Could you check a few things on this drawing? It's one solid part, dimensions in mm from its lowest x, y, z. Coordinates: 2 decimals unless noted, no trailing zeros. Order: outer loops, then holes, each group sorted by start corner. A loop starts at its lowest first (then second) coordinate and runs counter-clockwise, first axis right, second up.
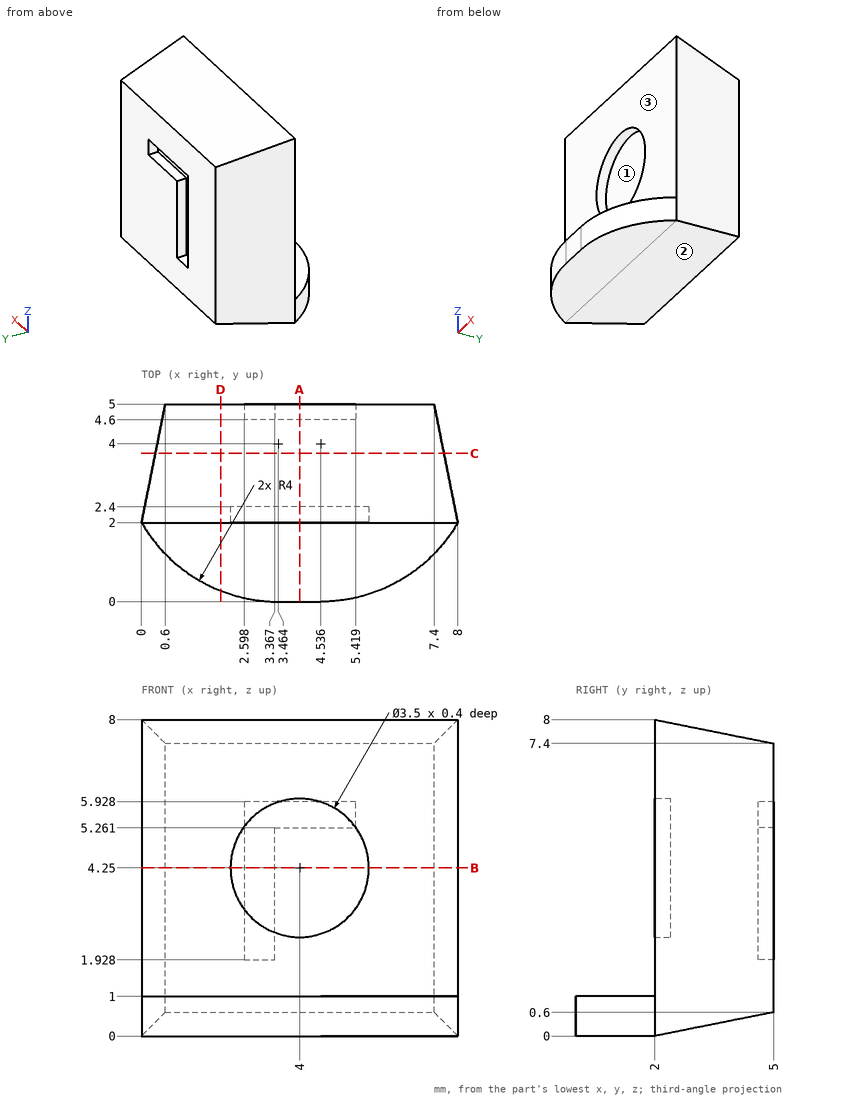
1. Imagine slicing it at A-A on x = 4. Please give me the cut outline in (y, z).
Completed:
outline: (0, 0) - (2, 0) - (5, 0.6) - (5, 5.26) - (4.6, 5.26) - (4.6, 5.93) - (5, 5.93) - (5, 7.4) - (2, 8) - (2, 6) - (2.4, 6) - (2.4, 2.5) - (2, 2.5) - (2, 1) - (0, 1) - close
2. I'm going to push flat-ended pins straight in: pin 1 (3 mm diameter, centred on x = 4, z = 4.25, fed in from -Y); pin 2 (3 mm diameter, centred on x = 3, z = 3.5, fed in from -Y); pin 3 (1 mm diameter, centred on y = 4, z = 4, fed in from -X). Where does each tip first touch, or does it pass through?
Completed:
pin 1: stops at y = 2.4
pin 2: stops at y = 2
pin 3: stops at x = 0.3
3. Imagine slicing it at D-D on x = 2. Please give me the cut outline in (y, z).
Completed:
outline: (0.28, 0) - (2, 0) - (5, 0.6) - (5, 7.4) - (2, 8) - (2, 1) - (0.28, 1) - close
4. Please list where these lines run through material, in increasing order: probe 1 along Y at (x, z) = (4.75, 3.75); probe 2 along Y at (x, z) = (1.25, 5); probe 3 along X at (y, z) = (2.1, 4.25).
Completed:
probe 1: y = 2.4 to 5
probe 2: y = 2 to 5
probe 3: x = 0.02 to 2.25, 5.75 to 7.98
5. Thinking about a two-plate mould opening in Z: for the marked faces 1, 2 and 3, which applies, pulls with the +Z half, pulls with the -Z half, needs draft (parallel to the pull), parting line crosses it, or undercut?
Completed:
face 1: undercut
face 2: pulls with the -Z half
face 3: needs draft
6. Imagine slicing it at B-B on z = 4.25. Please give me the cut outline in (x, y), then the cut area to 3 significant figures.
Completed:
outline: (0, 2) - (2.25, 2) - (2.25, 2.4) - (5.75, 2.4) - (5.75, 2) - (8, 2) - (7.4, 5) - (3.37, 5) - (3.37, 4.6) - (2.6, 4.6) - (2.6, 5) - (0.6, 5) - close
area: 20.5 mm2
7. Imagine slicing it at C-C on y = 3.75. Please give me the cut outline in (x, z), then the cut area to 3 significant figures.
Completed:
outline: (0.35, 0.35) - (7.65, 0.35) - (7.65, 7.65) - (0.35, 7.65) - close
area: 53.3 mm2
